Could you check a few things on this model? Use its own coordinates, in mm. Give positions to 0.01 mm unless a question says otherwise; leave off trailing zeros. Order: outer loops, then holes, each group sorted by start corner. A loop starts at its lowest first (then second) coordinate and runs counter-clockwise, first axis right, second up. Notation, with made-up numbers: (39, 9) -> (47, 9) arc R30 cw to (47, 38) -> close; hole circle Ø4 at (40, -31). An arc over 180 degrees is marked (long way). One line per item, written item: value.
```python
from build123d import *

# Parameters (mm, degrees)
MODEL_R             = 1.25
BOSS_EXTRUDE1_DEPTH = 3
SKETCH1_R           = 0.75
CUT_EXTRUDE1_DEPTH  = 10


with BuildPart() as part:
    # Model → Boss-Extrude1 (new body)
    with BuildSketch(Plane.XY):
        Polygon((41.057603072, 7.198758191), (141.057603072, 7.198758191), (161.057603072, 27.198758191), (161.057603072, 57.198758191), (171.057603072, 67.198758191), (171.057603072, 107.198758191), (161.057603072, 117.198758191), (161.057603072, 147.198758191), (141.057603072, 167.198758191), (41.057603072, 167.198758191), (21.057603072, 147.198758191), (21.057603072, 117.198758191), (11.057603072, 107.198758191), (11.057603072, 67.198758191), (21.057603072, 57.198758191), (21.057603072, 27.198758191), align=None)
        with Locations((133.557603072, 9.698758191)):
            Circle(MODEL_R, mode=Mode.SUBTRACT)
        with Locations((158.557603072, 34.698758191)):
            Circle(MODEL_R, mode=Mode.SUBTRACT)
        with Locations((149.289836119, 18.966525144)):
            Circle(MODEL_R, mode=Mode.SUBTRACT)
        with Locations((48.557603072, 9.698758191)):
            Circle(MODEL_R, mode=Mode.SUBTRACT)
        with Locations((23.557603072, 34.698758191)):
            Circle(MODEL_R, mode=Mode.SUBTRACT)
        with Locations((32.825370025, 18.966525144)):
            Circle(MODEL_R, mode=Mode.SUBTRACT)
        with Locations((133.557603072, 164.698758191)):
            Circle(MODEL_R, mode=Mode.SUBTRACT)
        with Locations((158.557603072, 139.698758191)):
            Circle(MODEL_R, mode=Mode.SUBTRACT)
        with Locations((149.289836119, 155.430991238)):
            Circle(MODEL_R, mode=Mode.SUBTRACT)
        with Locations((48.557603072, 164.698758191)):
            Circle(MODEL_R, mode=Mode.SUBTRACT)
        with Locations((23.557603072, 139.698758191)):
            Circle(MODEL_R, mode=Mode.SUBTRACT)
        with Locations((32.825370025, 155.430991238)):
            Circle(MODEL_R, mode=Mode.SUBTRACT)
        with Locations((17.825370025, 63.966525144)):
            Circle(MODEL_R, mode=Mode.SUBTRACT)
        with Locations((13.557603072, 87.198758191)):
            Circle(MODEL_R, mode=Mode.SUBTRACT)
        with Locations((17.825370025, 110.430991238)):
            Circle(MODEL_R, mode=Mode.SUBTRACT)
        with Locations((164.289836119, 63.966525144)):
            Circle(MODEL_R, mode=Mode.SUBTRACT)
        with Locations((168.557603072, 87.198758191)):
            Circle(MODEL_R, mode=Mode.SUBTRACT)
        with Locations((164.289836119, 110.430991238)):
            Circle(MODEL_R, mode=Mode.SUBTRACT)
    extrude(amount=BOSS_EXTRUDE1_DEPTH)

    # Sketch1 → Cut-Extrude1 (cut)
    with BuildSketch(Plane.XY.offset(3)):
        with Locations((91.057603072, 148.911555292)):
            Circle(SKETCH1_R)
        with Locations((37.612753044, 118.055156741)):
            Circle(SKETCH1_R)
        with Locations((144.502453099, 118.055156741)):
            Circle(SKETCH1_R)
        with Locations(Location((144.502453099, 56.342359641, 0), (0, 0, 180))):
            Circle(SKETCH1_R)
        with Locations(Location((91.057603072, 25.485961091, 0), (0, 0, 180))):
            Circle(SKETCH1_R)
        with Locations(Location((37.612753044, 56.342359641, 0), (0, 0, 180))):
            Circle(SKETCH1_R)
    extrude(amount=-CUT_EXTRUDE1_DEPTH, mode=Mode.SUBTRACT)


solid = part.part
```
1) Suppose I cut it at C-C, the plane x = 29. Write out the boundary of the cut face in (y, z), then the cut area to 3 significant figures.
Answer below:
outline: (19.26, 0) -> (155.14, 0) -> (155.14, 3) -> (19.26, 3) -> close
area: 408 mm2
2) For P1, Ø0.9, axis at y = 40.5, z = 1.5, coming from the -X side, with a flat end and sliding along its axis, tell me the tip position at first contact or that it passes through.
Answer below:
P1: stops at x = 21.06
3) Suppose I cut it at B-B, the plane z = 0.9. State how many separate pieces and enclosed holes the cut face has, then the cut area to 3 significant figures.
Answer below:
separate pieces: 1
enclosed holes: 24
area: 22,500 mm2
4) Suppose I cut it at A-A, the plane y = 43.5. Write out the boundary of the cut face in (x, z).
Answer below:
outline: (21.06, 0) -> (161.06, 0) -> (161.06, 3) -> (21.06, 3) -> close
5) If I drill on line 1 along X through (y, z) = (34, 0.55); line 2 along X through (y, z) = (147, 1.85); line 3 along Y through (x, z) = (159, 0.8), over which ranges is the centre line in solid material (lowest first)?
Answer below:
line 1: x = 21.06 to 22.52, 24.59 to 157.52, 159.59 to 161.06
line 2: x = 21.06 to 161.06
line 3: y = 25.14 to 33.53, 35.87 to 138.53, 140.87 to 149.26
